Here's the drawing with two shaded views (mm, measured from the low corner). I have some questions. A direction names the side the tool comes from. Give positions to 0.01 mm unless a question says otherwise; leave off trailing zeros. Write each loop counter-clockwise with the first axis right and the second up, starting at its lowest first coordinate (ties: lowest second). Pieces come first, ordered by that corner, then holes. Notation, with made-up numbers: (74.5, -25) -> (88.5, -25) arc R6 ccw to (88.5, -21) -> close; hole circle Ø11 at (72.25, 37.25). An arc over 180 degrees is marked (long way). Put each result on its own line as item: value. Start each with the question number.
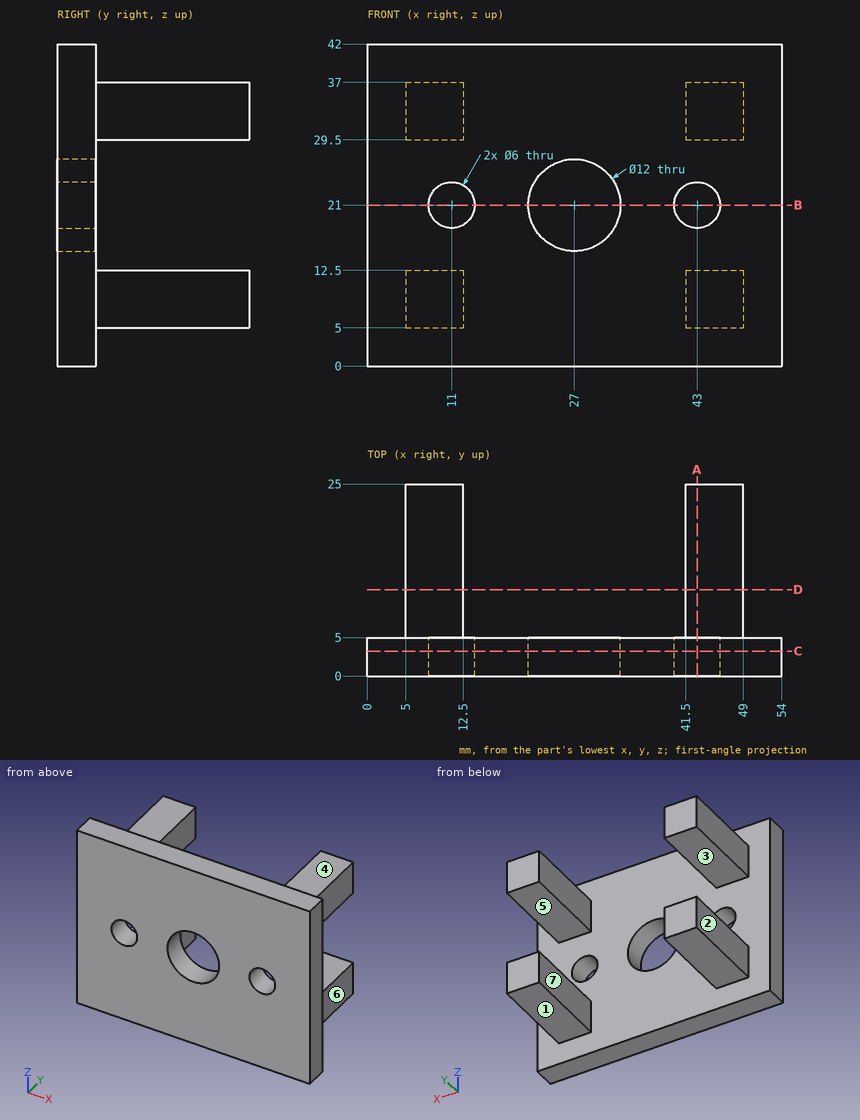
1) I want a section at C-C, the plane y = 3.25. Write out the boundary of the cut face in (x, z), and give its area (3 significant figures).
2) I'm going to push flat-ended pins straight in: pin 1 Ø1.5 at (x, z) = (23.5, 10.5) entering from +Y; pin 2 Ø6 at (x, y) = (9, 19) entering from -Z; pin 3 Ø5 at (y, z) = (18, 37.5) entering from +X. Where does each tip first touch, or does it pass through?
3) I want a section at B-B, the plane z = 21. Write out the boundary of the cut face in (x, y), and give its area (3 significant figures).
4) Which directions (+Z, -Z, +X, -X, +Y, -Y) give clear straight access to the entire face, cutting with the end or side of a thin tool? Please do the marked faces 4, 5, 6 and 7.
5) Thinking about a two-plate mould opening in Z: for the marked faces 1, 2 and 3, which applies, released by +Z, released by -Z, zero draft, split by the parting line, or undercut?
6) I want a section at D-D, the plane y = 11.25. Write out the boundary of the cut face in (x, z).
7) I want a section at A-A, the plane x = 43. Write out the boundary of the cut face in (y, z).
8) I need wall thicknesses on probe 1 along X at (y, z) = (1.75, 21); probe 2 along X at (y, z) = (11, 9); probe 3 along Z at (x, y) = (7.5, 23.25). Which ranges of each line are inside material? Lowest first, please.
Established:
1. outline: (0, 0) -> (54, 0) -> (54, 42) -> (0, 42) -> close; hole circle Ø6 at (11, 21); hole circle Ø12 at (27, 21); hole circle Ø6 at (43, 21)
1. area: 2,100 mm2
2. pin 1: stops at y = 5
2. pin 2: stops at z = 5
2. pin 3: stops at x = 49
3. outline: (0, 0) -> (8, 0) -> (8, 5) -> (0, 5) -> close; (14, 0) -> (21, 0) -> (21, 5) -> (14, 5) -> close; (33, 0) -> (40, 0) -> (40, 5) -> (33, 5) -> close; (46, 0) -> (54, 0) -> (54, 5) -> (46, 5) -> close
3. area: 150 mm2
4. face 4: +Z, +X, -X, +Y
4. face 5: +X, -X, +Y
4. face 6: +Z, -Z, +X, +Y
4. face 7: +Z, -Z, +Y
5. face 1: released by -Z
5. face 2: zero draft
5. face 3: undercut
6. outline: (5, 5) -> (12.5, 5) -> (12.5, 12.5) -> (5, 12.5) -> close; (5, 29.5) -> (12.5, 29.5) -> (12.5, 37) -> (5, 37) -> close; (41.5, 5) -> (49, 5) -> (49, 12.5) -> (41.5, 12.5) -> close; (41.5, 29.5) -> (49, 29.5) -> (49, 37) -> (41.5, 37) -> close
7. outline: (0, 0) -> (5, 0) -> (5, 5) -> (25, 5) -> (25, 12.5) -> (5, 12.5) -> (5, 18) -> (0, 18) -> close; (0, 24) -> (5, 24) -> (5, 29.5) -> (25, 29.5) -> (25, 37) -> (5, 37) -> (5, 42) -> (0, 42) -> close
8. probe 1: x = 0 to 8, 14 to 21, 33 to 40, 46 to 54
8. probe 2: x = 5 to 12.5, 41.5 to 49
8. probe 3: z = 5 to 12.5, 29.5 to 37
